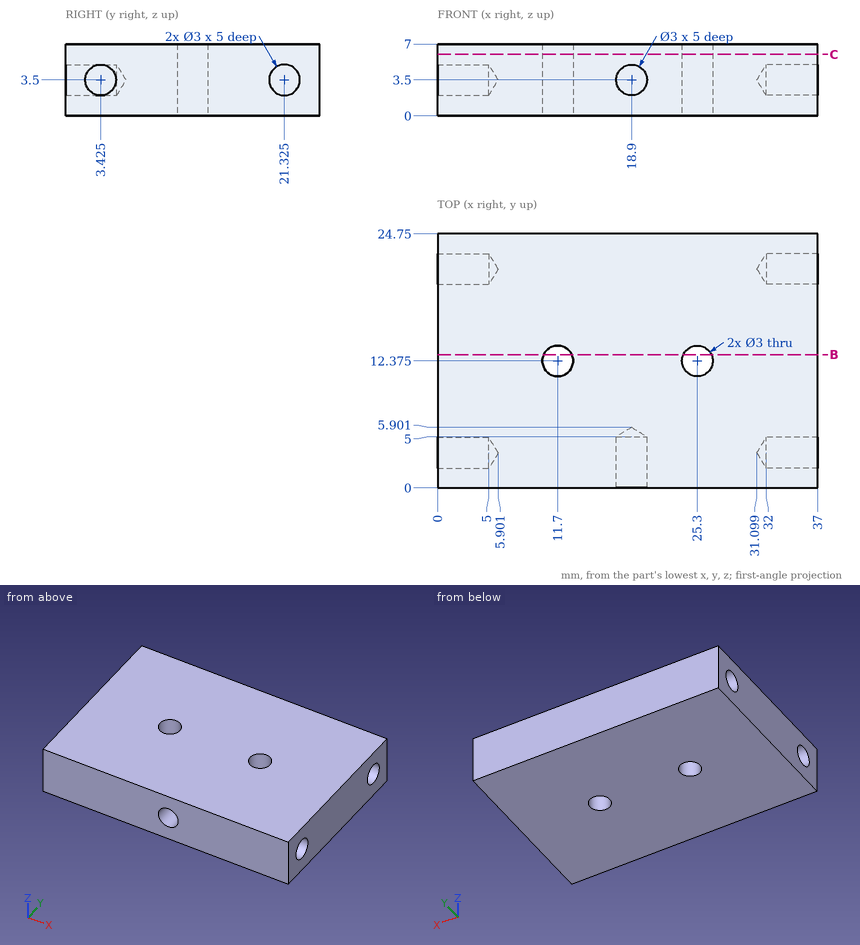
Here's the drawing with two shaded views (mm, measured from the low corner). I have some questions. Give positions to 0.01 mm unless a question says otherwise; leave off trailing zeros. Order: outer loops, then holes, each group sorted by start corner. A loop starts at its lowest first (then second) coordinate and runs counter-clockwise, first axis right, second up.
Q1. Suppose I cut it at C-C, the plane z = 6. Count the separate pieces of the cut face and the enclosed holes in it, and give its area (3 significant figures).
Q2. I'm going to push flat-ended pins straight in: P1, Ø12, axis at x = 32, y = 13, coming from the -Z side; P2, Ø2.5, axis at y = 3.425, z = 3.5, coming from the +X side. Where does each tip first touch, or does it pass through?
Q3. Suppose I cut it at B-B, the plane y = 13. Write out the boundary of the cut face in (x, z), and give its area (3 significant figures).
Q4. If I drill on line 1 along X through (y, z) = (1.7, 3.5); line 2 along X through (y, z) = (13, 2.5); line 3 along X through (y, z) = (13.75, 1.75), over which ranges is the centre line in solid material (lowest first)?
Solution:
1. separate pieces: 1
1. enclosed holes: 2
1. area: 902 mm2
2. P1: stops at z = 0
2. P2: stops at x = 31.85
3. outline: (0, 0) - (10.34, 0) - (10.34, 7) - (0, 7) - close; (13.06, 0) - (23.94, 0) - (23.94, 7) - (13.06, 7) - close; (26.66, 0) - (37, 0) - (37, 7) - (26.66, 7) - close
3. area: 221 mm2
4. line 1: x = 0 to 17.4, 20.4 to 37
4. line 2: x = 0 to 10.34, 13.06 to 23.94, 26.66 to 37
4. line 3: x = 0 to 11.1, 12.3 to 24.7, 25.9 to 37
